Print and shaded views of the part. All mm, measured from the part's lowest x, y and z. Round coordinates to 2 decimals unless told otherwise and drop trailing zeros. Loops run counter-clockwise (first coordinate to the right, second up) from the corner with the lowest first, then second, coordinate; pieces in that order, holes last. Notation, with made-up numbers: (4, -28.5) -> (21, -28.5) arc R23 ccw to (21, -16.5) -> close; hole circle Ø5 at (14.25, 85). An arc over 180 degrees is marked (long way). Use a Markdown table: item, result.
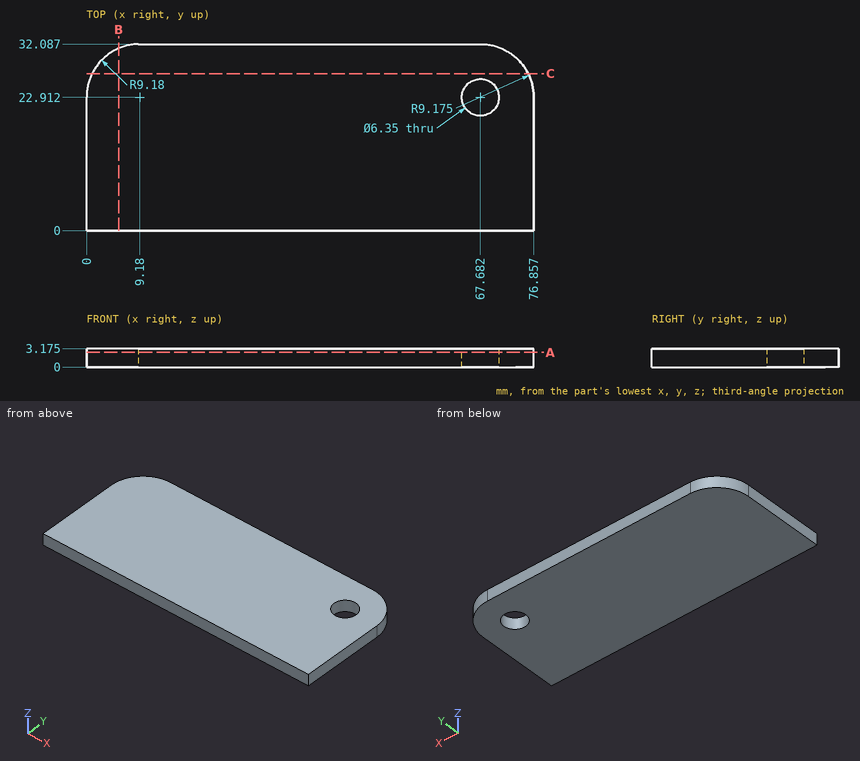
Q1. Drill centre lines: L1, parallel to X at y = 21, z = 2.4; L2, parallel to Y at x = 70.5, z = 2.3; L3, parallel to X at y = 24.5, z = 0.9. Where is each one in solid material? Low to high. Write a range as from..to.
Results list:
| item | result |
|---|---|
| L1 | x = 0..65.15, 70.22..76.86 |
| L2 | y = 0..21.45, 24.37..31.64 |
| L3 | x = 0.14..64.93, 70.43..76.72 |
Q2. Band-saw the part on B-B, the plane x = 5.5. Give the cut face in (y, z) (3 decimals).
Results list:
| item | result |
|---|---|
| outline | (0, 0) -> (31.322, 0) -> (31.322, 3.175) -> (0, 3.175) -> close |
Q3. Band-saw the part on C-C, the plane y = 27. Give the cut face in (x, z) (3 decimals), plus the area to 3 significant figures.
Results list:
| item | result |
|---|---|
| outline | (0.96, 0) -> (75.896, 0) -> (75.896, 3.175) -> (0.96, 3.175) -> close |
| area | 238 mm² |
Q4. Flat gauge pin, fed straight in: pin 1 (6 mm diameter, centred on x = 55.5, y = 10.5, fed in from -Z). Where does the tip first touch, or does it go through?
Results list:
| item | result |
|---|---|
| pin 1 | stops at z = 0 |
Q5. Band-saw the part on A-A, the plane z = 2.55. Give the cut face in (x, y) (3 decimals), plus the area to 3 significant figures.
Results list:
| item | result |
|---|---|
| outline | (0, 0) -> (76.857, 0) -> (76.857, 22.912) arc R9.175 ccw to (67.682, 32.087) -> (8.877, 32.087) arc R9.18 ccw to (0, 22.912) -> close; hole circle Ø6.35 at (67.682, 22.912) |
| area | 2,400 mm² |
